The model under review builds one solid part; all positions refer to its coordinate system, in mm. Face numbers are marked on the shaded views. A direction names the side the tool comes from. Give positions to 0.01 mm unless a question says otherwise; leave off trailing zeros. Order: outer loops, then holes, each group sorted by start corner. A loop starts at its lowest first (then second) coordinate and runs counter-clockwise, first axis right, second up. Notation, with made-up numbers: M -31.5,73 L 4.5,73 A16 ccw 4.5,98 Z; hole C -2.5,-33 d9. An arc over 180 degrees is marked long. One line per question, with ' | ' between items. Start each with the question number.
1. We need section A-A on y = 5.5. Write out the cut boundary in (x, z), then the cut area to 3 significant figures.
2. We need section B-B on x = 348.5. Write out the cut boundary in (y, z).
3. We need section C-C on z = 101.5. Write out the cut boundary in (x, y).
4. Insertion check: P1, Ø1, axis at y = 164.5, z = -93, coming from the +X side. The pin has a flat end and moves straight along its axis. Give the tip position at first contact, or say it passes through.
5. We need section D-D on x = -312.5. Write out the cut boundary in (y, z).
6. For the marked faces 4, 5 and 6, list the 3-axis set-ups (+Z, -Z, +X, -X, +Y, -Y) from which the entire face can be reached by the end or side of a thin tool; tool diameter is ignored.
7. Wall thickness on L1, parallel to Z at x = 357.5, y = 12; L2, parallel to X at y = -34, z = 87.5; L3, parallel to Y at x = 246, z = -99.5: over which ranges is each line inside the solid? List them lowest first.
8. The part is to be moulded in two halves that separate along Z. For the marked faces 1, 2 and 3, say which applies: +Z half, -Z half, draft (parallel to the pull), parting line (faces both ways), or undercut.
```python
from build123d import *

# Parameters (mm, degrees)
BOSS_EXTRUDE1_DEPTH = 158.75
SKETCH2_W           = 279.4
SKETCH2_H           = 266.7
CUT_EXTRUDE1_DEPTH  = 139.7
FILLET1_R           = 10.16


with BuildPart() as part:
    # Sketch1 → Boss-Extrude1 (new, symmetric)
    with BuildSketch(Plane.XY):
        Polygon((-406.4, 88.9), (-406.4, -88.9), (406.4, -88.9), (406.4, 88.9), (76.2, 88.9), (76.2, 215.9), (-126.973642647, 215.9), (-215.9, 88.9), align=None)
    extrude(amount=BOSS_EXTRUDE1_DEPTH, both=True)

    # Sketch2 → Cut-Extrude1 (cut)
    with BuildSketch(Plane(origin=(0, 88.9, 0), x_dir=(1, 0, 0), z_dir=(0, 1, 0))):
        with Locations((241.3, 0)):
            Rectangle(SKETCH2_W, SKETCH2_H)
    extrude(amount=-CUT_EXTRUDE1_DEPTH, mode=Mode.SUBTRACT)

    # Fillet1
    fillet1_edges = [part.edges().sort_by_distance(p)[0] for p in [
        (406.4, 0, -158.75),
        (-406.4, 0, -158.75),
        (-311.15, 88.9, -158.75),
        (-215.9, 88.9, 0),
        (-126.973642647, 215.9, 0),
        (76.2, 215.9, 0),
        (76.2, 88.9, 0),
        (406.4, 88.9, 0),
        (-406.4, 88.9, 0),
        (406.4, 0, 158.75),
        (241.3, 88.9, 158.75),
        (76.2, 152.4, 158.75),
        (101.6, -50.8, 0),
        (101.6, 19.05, 133.35),
        (241.3, -50.8, -133.35),
        (101.6, 19.05, -133.35),
        (381, -50.8, 0),
        (241.3, -50.8, 133.35),
        (-25.386821324, 215.9, 158.75),
        (381, 19.05, 133.35),
        (101.6, 88.9, 0),
        (241.3, 88.9, 133.35),
        (381, 88.9, 0),
        (241.3, 88.9, -133.35),
        (-171.436821324, 152.4, 158.75),
        (-311.15, 88.9, 158.75),
        (-171.436821324, 152.4, -158.75),
        (-406.4, 0, 158.75),
        (-25.386821324, 215.9, -158.75),
        (76.2, 152.4, -158.75),
        (241.3, 88.9, -158.75),
    ]]
    fillet(fillet1_edges, radius=FILLET1_R)


solid = part.part
```
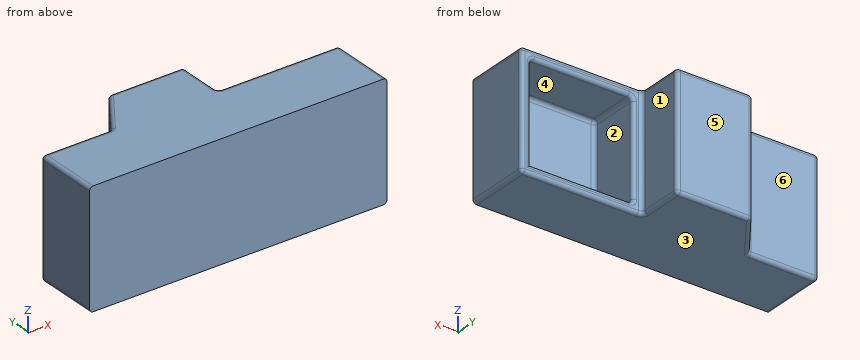
Entries:
1) outline: M -406.4,-148.59 A10.16 ccw -396.24,-158.75 L 396.24,-158.75 A10.16 ccw 406.4,-148.59 L 406.4,148.59 A10.16 ccw 396.24,158.75 L -396.24,158.75 A10.16 ccw -406.4,148.59 Z; hole M 101.6,-123.19 A10.16 ccw 111.76,-133.35 L 381,-133.35 L 381,123.19 A10.16 ccw 370.84,133.35 L 111.76,133.35 A10.16 ccw 101.6,123.19 Z | area: 184,000 mm^2
2) outline: M -88.9,-158.75 L 78.74,-158.75 A10.16 ccw 88.9,-148.59 L 88.9,-143.51 A10.16 ccw 78.74,-133.35 L -40.64,-133.35 A10.16 cw -50.8,-123.19 L -50.8,123.19 A10.16 cw -40.64,133.35 L 78.74,133.35 A10.16 ccw 88.9,143.51 L 88.9,148.59 A10.16 ccw 78.74,158.75 L -88.9,158.75 Z
3) outline: M -406.4,-88.9 L 406.4,-88.9 L 406.4,78.74 A10.16 ccw 396.24,88.9 L 391.16,88.9 A10.16 ccw 381,78.74 L 381,-40.64 A10.16 cw 370.84,-50.8 L 111.76,-50.8 A10.16 cw 101.6,-40.64 L 101.6,78.74 A10.16 ccw 91.44,88.9 L 86.36,88.9 A10.16 cw 76.2,99.06 L 76.2,205.74 A10.16 ccw 66.04,215.9 L -121.68,215.9 A10.16 ccw -130.01,211.57 L -212.87,93.23 A10.16 cw -221.19,88.9 L -396.24,88.9 A10.16 ccw -406.4,78.74 Z
4) P1: stops at x = 76.2
5) outline: M -88.9,-158.75 L 78.74,-158.75 A10.16 ccw 88.9,-148.59 L 88.9,148.59 A10.16 ccw 78.74,158.75 L -88.9,158.75 Z
6) face 4: +Y | face 5: +Z, -Z, +X, -X, +Y | face 6: +Z, -Z, -X, +Y
7) L1: z = -158.75 to -133.35, 133.35 to 158.75 | L2: x = -406.4 to 101.6, 381 to 406.4 | L3: y = -88.9 to -50.8
8) face 1: draft | face 2: undercut | face 3: -Z half
